```python
from build123d import *

# Parameters (mm, degrees)
F0_R      = 1
F0_R_2    = 1.25
F0_R_3    = 4.2
F0_R_4    = 1.275
F0_W      = 11.2
F0_H      = 6.2
F1_DEPTH  = 3
F0_W_2    = 110
F0_H_2    = 130
F2_DEPTH  = 3
F3_DEPTH  = 6
F5_DEPTH  = 45
F7_DEPTH  = 60
F9_DEPTH  = 40
F11_DEPTH = 21


with BuildPart() as f1:
    # F0 (on Top) → F1 (new body)
    with BuildSketch(Plane.XY):
        with BuildLine():
            ThreePointArc((26.3367733861, -20), (31.3415301151, -10.5514985873), (33.0700110734, 0))
            ThreePointArc((33.0700110734, 0), (14.7007722744, 29.6228446799), (-20, 26.3367733861))
            Line((-20, 26.3367733861), (-20, -20))
            Line((-20, -20), (26.3367733861, -20))
        make_face()
        with Locations((-15, 3.4738e-06)):
            Circle(F0_R, mode=Mode.SUBTRACT)
        Circle(F0_R_2, mode=Mode.SUBTRACT)
        with Locations((-7.68e-08, 19)):
            Circle(F0_R_3, mode=Mode.SUBTRACT)
        with Locations((0, 28.25)):
            Circle(F0_R_4, mode=Mode.SUBTRACT)
        with Locations((11.580758131, 16.0824482103)):
            Rectangle(F0_W, F0_H, mode=Mode.SUBTRACT)
        with Locations((28.25, 0)):
            Circle(F0_R_4, mode=Mode.SUBTRACT)
        with BuildLine():
            Line((-20, -20), (-20, 26.3367733861))
            ThreePointArc((-20, 26.3367733861), (-23.3840290839, -23.3840290839), (26.3367733861, -20))
            Line((26.3367733861, -20), (-20, -20))
        make_face()
        with Locations((-28.25, 0)):
            Circle(F0_R_4, mode=Mode.SUBTRACT)
    extrude(amount=-F1_DEPTH)

    # F0 (on Top) → F2 (join)
    with BuildSketch(Plane.XY):
        with Locations((20, 30)):
            Rectangle(F0_W_2, F0_H_2)
        with BuildLine():
            ThreePointArc((26.3367733861, -20), (-23.3840290839, -23.3840290839), (-20, 26.3367733861))
            Line((-20, 26.3367733861), (-20, 80))
            Line((-20, 80), (60, 80))
            Line((60, 80), (60, -20))
            Line((60, -20), (26.3367733861, -20))
        make_face(mode=Mode.SUBTRACT)
        with BuildLine():
            ThreePointArc((26.3367733861, -20), (31.3415301151, -10.5514985873), (33.0700110734, 0))
            ThreePointArc((33.0700110734, 0), (14.7007722744, 29.6228446799), (-20, 26.3367733861))
            Line((-20, 26.3367733861), (-20, -20))
            Line((-20, -20), (26.3367733861, -20))
        make_face()
        with Locations((-15, 3.4738e-06)):
            Circle(F0_R, mode=Mode.SUBTRACT)
        Circle(F0_R_2, mode=Mode.SUBTRACT)
        with Locations((-7.68e-08, 19)):
            Circle(F0_R_3, mode=Mode.SUBTRACT)
        with Locations((0, 28.25)):
            Circle(F0_R_4, mode=Mode.SUBTRACT)
        with Locations((11.580758131, 16.0824482103)):
            Rectangle(F0_W, F0_H, mode=Mode.SUBTRACT)
        with Locations((28.25, 0)):
            Circle(F0_R_4, mode=Mode.SUBTRACT)
        with BuildLine():
            Line((-20, -20), (-20, 26.3367733861))
            ThreePointArc((-20, 26.3367733861), (-23.3840290839, -23.3840290839), (26.3367733861, -20))
            Line((26.3367733861, -20), (-20, -20))
        make_face()
        with Locations((-28.25, 0)):
            Circle(F0_R_4, mode=Mode.SUBTRACT)
        with BuildLine():
            ThreePointArc((-20, 26.3367733861), (14.7007722744, 29.6228446799), (33.0700110734, 0))
            ThreePointArc((33.0700110734, 0), (31.3415301151, -10.5514985873), (26.3367733861, -20))
            Line((26.3367733861, -20), (60, -20))
            Line((60, -20), (60, 80))
            Line((60, 80), (-20, 80))
            Line((-20, 80), (-20, 26.3367733861))
        make_face()
        with Locations((-15, 3.4738e-06)):
            Circle(F0_R)
        Circle(F0_R_2)
    extrude(amount=F2_DEPTH)

    # F0 (on Top) → F3 (join)
    with BuildSketch(Plane.XY):
        with Locations((-15, 3.4738e-06)):
            Circle(F0_R)
    extrude(amount=-F3_DEPTH)

    # F4 (on face) → F5 (cut)
    with BuildSketch(Plane.XZ.offset(35)):
        Polygon((1, 3), (-1, 3), (0, 1), align=None)
    extrude(amount=-F5_DEPTH, mode=Mode.SUBTRACT)

    # F6 (on face) → F7 (cut)
    with BuildSketch(Plane(origin=(0, 95, 0), x_dir=(-1, 0, 0), z_dir=(0, 1, 0))):
        Polygon((-1, 3), (0, 1), (1, 3), align=None)
    extrude(amount=-F7_DEPTH, mode=Mode.SUBTRACT)

    # F8 (on face) → F9 (cut)
    with BuildSketch(Plane.YZ.offset(75)):
        Polygon((1, 3), (-1, 3), (0, 1), align=None)
    extrude(amount=-F9_DEPTH, mode=Mode.SUBTRACT)

    # F10 (on Right) → F11 (cut, symmetric)
    with BuildSketch(Plane.YZ):
        Polygon((-1, 3), (0, 1), (1, 3), align=None)
    extrude(amount=F11_DEPTH, both=True, mode=Mode.SUBTRACT)


solid = f1.part
```
The listing builds one solid part. Answer for the finished solid, in the listing's coordinates (mm). A direction names the side the tool comes from. Give positions to 0.01 mm unless a question says otherwise; leave off trailing zeros. Order: outer loops, then holes, each group sorted by start corner. A loop starts at its lowest first (then second) coordinate and runs counter-clockwise, first axis right, second up. Notation, with made-up numbers: (74.5, -18.75) - (114.5, -18.75) arc R34 cw to (114.5, 13.25) - close; hole circle Ø8 at (-16, -25.5). An arc over 180 degrees is marked (long way). Use one line per item in the form item = value. Start each with the question number.
(1) The mould has two halves that part along X. Classify faces 3 (the flat face through (-35, 29, 1)), 4 (the flat face through (31, 45, 0)), 5 (the flat face through (75, 29, 1)), 6 (the flat face through (12, 19.182, 0)): released by +X, released by -X, zero draft, split by the parting line, or undercut.
(2) A cutting plane is placed at A-A, the plane y = 80. Write down the section's boundary in (x, z).
(3) Flat-ended cylindrical pins translate along their axes: pin 1 Ø3 at (x, y) = (-0.5, 0) entering from -Z; pin 2 Ø5 at (x, z) = (60, -3) entering from -Y; pin 3 Ø10 at (x, y) = (44.5, 38.5) entering from -Z; pin 4 Ø5 at (y, z) = (13.5, -4.5) entering from -X. Find the tip coordinate at first contact, or state that the pin passes through.
(4) A cutting plane is placed at D-D, the plane y = 5.5. Write down the section's boundary in (x, z), then the cut area to 3 significant figures.
(5) Consider line 1 (Y direction, x = 0, z = -0.55) (3 decimals); line 2 (Y direction, x = -28.25, z = 0.5) (3 decimals); line 3 (X direction, y = 18.5, z = -0.75). Determine where each line is inside the solid, lowest interval first. Write a range as from..to.
(6) A cutting plane is placed at C-C, the plane y = -17. Write down the section's boundary in (x, z), then the cut area to 3 significant figures.
(7) A cutting plane is placed at B-B, the plane y = 31. Write down the section's boundary in (x, z), then the cut area to 3 significant figures.
(8) For faces 1 (the flat face through (5.981, 16, 0)), 2 (the flat face through (19, 31, 3)), determine the directions among +Z, -Z, +X, -X, +Y, -Y from which every point of the face is accessible in a straight line to the end or side of a thin tool.
Ans:
q1.face_3 = released by -X
q1.face_4 = zero draft
q1.face_5 = released by +X
q1.face_6 = undercut
q2.outline = (-35, 0) - (75, 0) - (75, 3) - (1, 3) - (0, 1) - (-1, 3) - (-35, 3) - close
q3.pin_1 = -3
q3.pin_2 = through
q3.pin_3 = 0
q3.pin_4 = -31.01
q4.outline = (-35, 0) - (-32.61, 0) - (-32.61, -3) - (32.61, -3) - (32.61, 0) - (75, 0) - (75, 3) - (1, 3) - (0, 1) - (-1, 3) - (-35, 3) - close
q4.area = 524 mm^2
q5.line_1 = -33.07..-1.25, 1.25..14.8, 23.2..26.975, 29.525..33.07
q5.line_2 = -35..-1.275, 1.275..95
q5.line_3 = -27.41..-4.17, 4.17..5.98, 17.18..27.41
q6.outline = (-35, 0) - (-28.37, 0) - (-28.37, -3) - (28.37, -3) - (28.37, 0) - (75, 0) - (75, 3) - (1, 3) - (0, 1) - (-1, 3) - (-35, 3) - close
q6.area = 498 mm^2
q7.outline = (-35, 0) - (-11.52, 0) - (-11.52, -3) - (11.52, -3) - (11.52, 0) - (75, 0) - (75, 3) - (-35, 3) - close
q7.area = 399 mm^2
q8.face_1 = +Z, -Z
q8.face_2 = +Z, +X, -X, +Y, -Y
